The drawing under review shows one solid part. Ordinate dimensions are in mm from its lowest x, y, z. A direction names the side the tool comes from. Give positions to 0.01 mm unless a question says otherwise; leave off trailing zeros. Order: outer loops, then holes, each group sorted by start corner. A loop starts at its lowest first (then second) coordinate and runs counter-clockwise, first axis right, second up. Notation, with made-up numbers: (-25, -22.75) -> (4, -22.75) arc R15 cw to (4, 1.25) -> close; hole circle Ø1 at (48.5, 63). An arc over 180 degrees is marked (long way). One line per item, written item: value. Start each with the question number.
1) Consider section A-A (x = 49.5). State the section outline as (y, z) points (1 decimal), plus the area to 3 significant figures.
2) Wall thickness on line 1 along Y through (x, z) = (34.5, 28.5); line 2 along Y through (x, z) = (35, 37); line 3 along X through (y, z) = (23, 41.5): over which ranges is each line inside the solid? List them lowest first. Write a range as from..to.
3) For pin 1 (16.5 mm diameter, centred on x = 47, z = 46.5, fed in from +Y); pin 2 (1.5 mm diameter, centred on x = 25, z = 14, fed in from -Y); pin 3 (6.5 mm diameter, centred on x = 38, y = 32.5, fed in from +Z); pin 4 (10 mm diameter, centred on y = 20.5, z = 58, fed in from -X), all flat-tipped, find the tip position at first contact; note any pin that passes through.
4) Consider section D-D (z = 12.7). State the section outline as (x, y) points, plus the area to 3 significant figures.
5) The part is to be moulded in two halves that separate along Z. For the marked faces 3, 4, 5 and 6, say which applies: released by +Z, released by -Z, zero draft, split by the parting line, or undercut.
6) Tool access review of the marked faces 1 and 2: name each direction out of +Z, -Z, +X, -X, +Y, -Y from which nothing blocks a thin tool from reaching the whole face with its end or side.
7) Consider section B-B (y = 43). State how many separate pieces and enclosed holes the cut face has, plus the area to 3 significant figures.
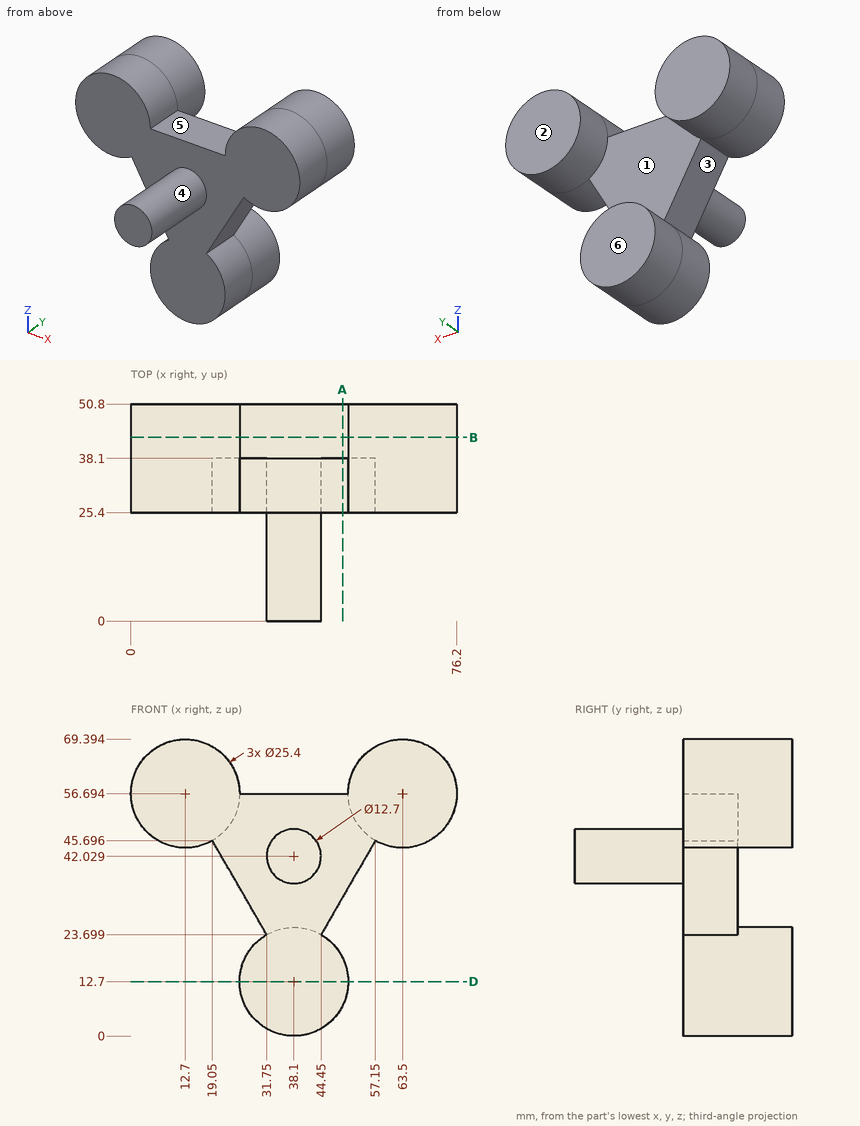
Checked values:
1. outline: (25.4, 7.1) -> (50.8, 7.1) -> (50.8, 18.3) -> (25.4, 18.3) -> close; (25.4, 32.4) -> (38.1, 32.4) -> (38.1, 56.7) -> (25.4, 56.7) -> close
1. area: 592 mm^2
2. line 1: y = 25.4..38.1
2. line 2: y = 0..38.1
2. line 3: x = 31.77..44.43
3. pin 1: stops at y = 50.8
3. pin 2: stops at y = 25.4
3. pin 3: stops at z = 56.69
3. pin 4: stops at x = 0
4. outline: (25.4, 25.4) -> (50.8, 25.4) -> (50.8, 50.8) -> (25.4, 50.8) -> close
4. area: 645 mm^2
5. face 3: undercut
5. face 4: split by the parting line
5. face 5: released by +Z
5. face 6: zero draft
6. face 1: +Y
6. face 2: +Z, -Z, +X, -X, +Y
7. separate pieces: 3
7. enclosed holes: 0
7. area: 1,520 mm^2
